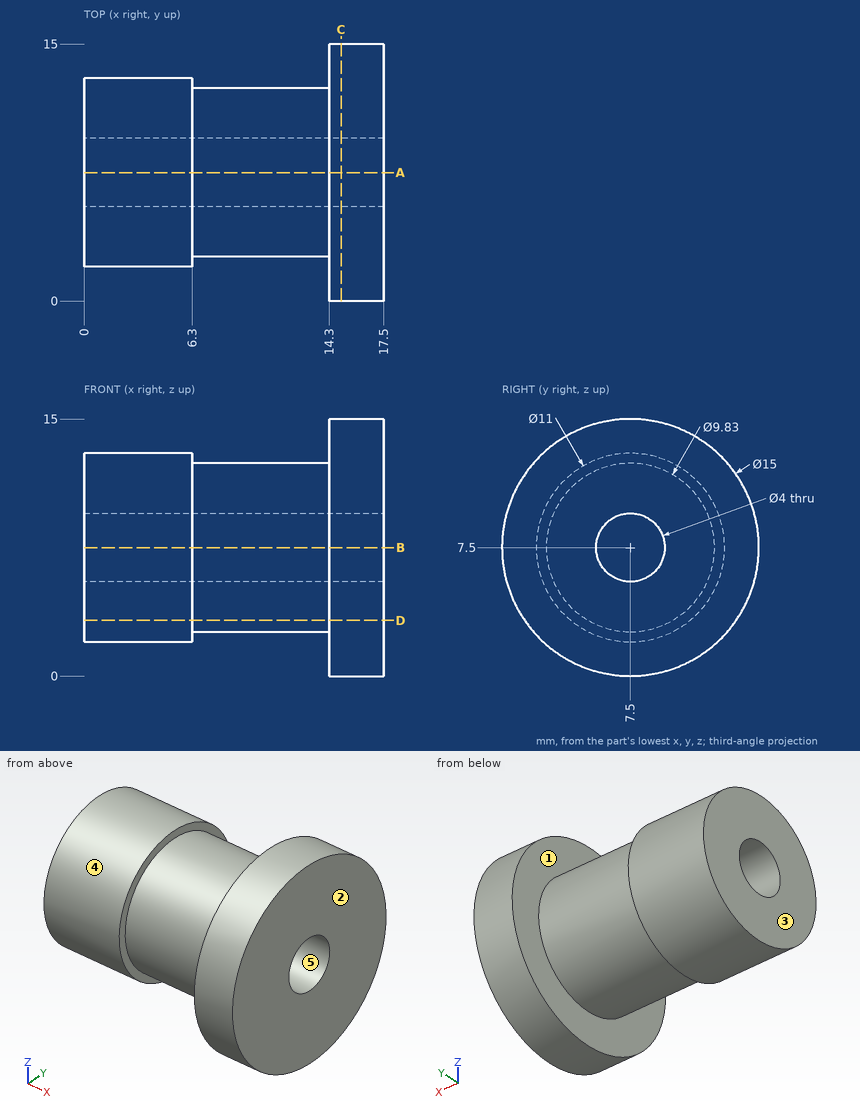
Print and shaded views of the part. All mm, measured from the part's lowest x, y and z. A direction names the side the tool comes from. Coordinates: 2 decimals unless noted, no trailing zeros. Loops run counter-clockwise (first coordinate to the right, second up) from the corner with the lowest first, then second, coordinate; pieces in that order, holes last. Notation, with made-up numbers: M 61.5,-23.5 L 83.5,-23.5 A23 cw 83.5,-6.5 Z; hole C -21,25 d4. An arc over 180 degrees is marked long. Use a Markdown table: item, result. Add a question column.
Q1. Probe L1, parallel to Y at x = 12.75, z = 7.5 (3 decimals); L2, parallel to Y at x = 3, z = 7.75; L3, parallel to X at y = 1.5, z = 10. List the from-to ranges inside material, lowest first.
Q2. Mould opens along Y. For the marked faces 3, 4 and 5 say: +Y half, -Y half, draft (parallel to the pull), parting line (faces both ways), or undercut.
Q3. Cut at D-D (z = 3.25). Write the cut outline in (x, y).
Q4. Cut at C-C (x = 15). Write the cut outline in (y, z), and give its area (3 significant figures).
Q5. Pin check, flat tips, straight feed: P1, Ø3, axis at x = 11, z = 9.5, coming from the -Y side; P2, Ø1.5, axis at x = 4, y = 8, coming from the -Z side; P3, Ø8, axis at x = 6.5, z = 8.5, coming from the +Y side. Stop position of each tip, or through.
Q6. Which spindle directions (+Z, -Z, +X, -X, +Y, -Y) get a long thin tool onto all of the face, cutting with end or side? Do the marked faces 1 and 2. Say none if no direction does.
Q7. Cut at A-A (y = 7.5). Write the cut outline in (x, z) (3 decimals), and give its area (3 significant figures).
Worked out:
| question | item | result |
|---|---|---|
| 1 | L1 | y = 2.585 to 5.5, 9.5 to 12.415 |
| 1 | L2 | y = 2.01 to 5.52, 9.48 to 12.99 |
| 1 | L3 | x = 14.3 to 17.5 |
| 2 | face 3 | draft |
| 2 | face 4 | parting line |
| 2 | face 5 | undercut |
| 3 | outline | M 0,4.01 L 6.3,4.01 L 6.3,5.03 L 14.3,5.03 L 14.3,1.32 L 17.5,1.32 L 17.5,13.68 L 14.3,13.68 L 14.3,9.97 L 6.3,9.97 L 6.3,10.99 L 0,10.99 Z |
| 4 | outline | C 7.5,7.5 d15; hole C 7.5,7.5 d4 |
| 4 | area | 164 mm2 |
| 5 | P1 | stops at y = 2.61 |
| 5 | P2 | stops at z = 2 |
| 5 | P3 | stops at y = 13 |
| 6 | face 1 | none |
| 6 | face 2 | +Z, -Z, +X, +Y, -Y |
| 7 | outline | M 0,2 L 6.3,2 L 6.3,2.585 L 14.3,2.585 L 14.3,0 L 17.5,0 L 17.5,5.5 L 0,5.5 Z; M 0,9.5 L 17.5,9.5 L 17.5,15 L 14.3,15 L 14.3,12.415 L 6.3,12.415 L 6.3,13 L 0,13 Z |
| 7 | area | 126 mm2 |
